Source: three-view drawing plus pictorial views. Frame: mm from the lowest corner of the part. A direction names the side the tool comes from. Round coordinates to 2 decimals unless told otherwise and drop trailing zeros. Write each loop counter-clockwise with the first axis right and the second up, starting at its lowest first coordinate (ties: lowest second). Pieces come first, ordered by that corner, then holes.
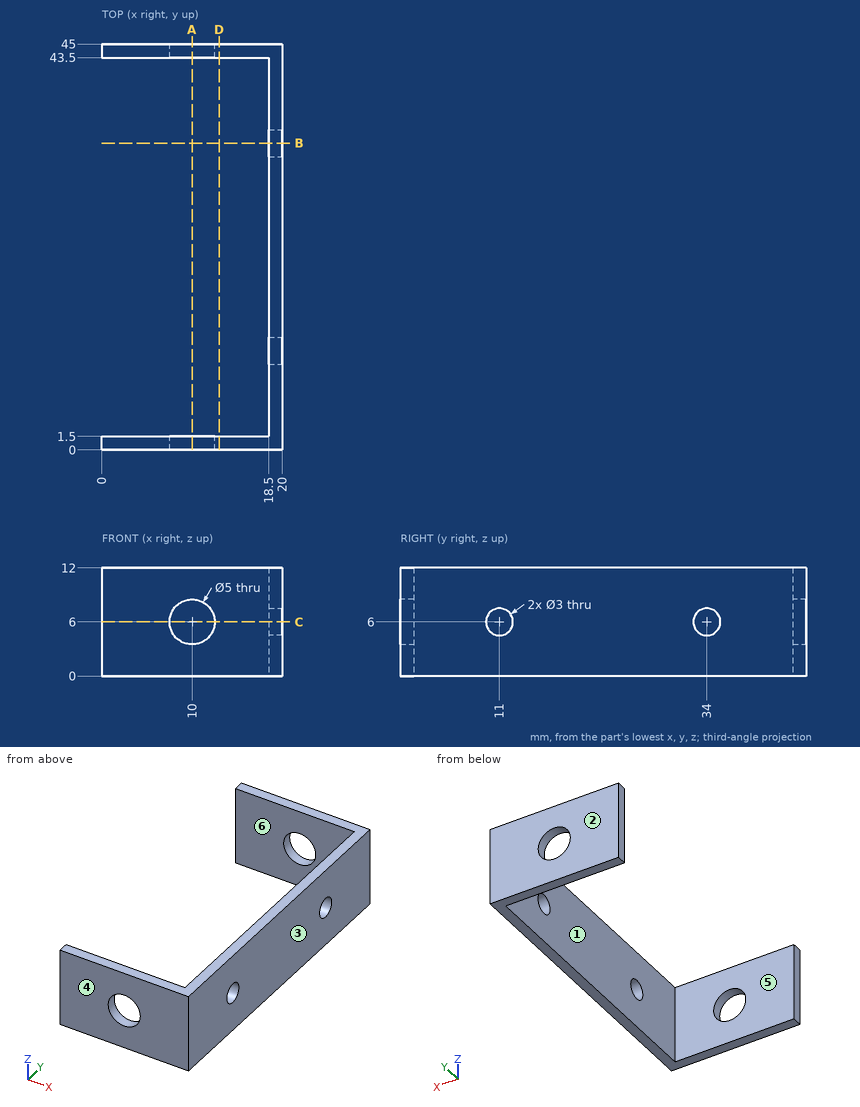
1) Draft query along Y for the marked faces 3, 4, 5 and 6. Return one class per face: pulls with the +Y half, pulls with the -Y half, needs draft (parallel to the pull), parting line crosses it, or undercut.
2) Section C-C on z = 6. Output: boundary loops of the cut face in (x, y), plus the area to 3 significant figures.
3) First-contact query: P1, Ø3.5, axis at y = 13, z = 7, coming from the -X side. Flat tip, straight axial feed; report the tip coordinate or a pass-through.
4) Section A-A on x = 10. Output: boundary loops of the cut face in (y, z).
5) Reachability of the marked faces 1 and 2 from +Z, -Z, +X, -X, +Y, -Y: full face, straight path, thin tool, end or side. Return the list, or none.
6) Line query: probe 1 along Y at (x, z) = (19.6, 6); probe 2 along Y at (x, z) = (8, 0.75); probe 3 along X at (y, z) = (0.5, 6). Output: solid intervals per line, ascending.
7) Section D-D on x = 13. Output: boundary loops of the cut face in (y, z).
8) Section B-B on y = 34. Output: boundary loops of the cut face in (x, z).
Filled in:
1. face 3: needs draft
1. face 4: pulls with the -Y half
1. face 5: undercut
1. face 6: undercut
2. outline: (0, 0) - (7.5, 0) - (7.5, 1.5) - (0, 1.5) - close; (0, 43.5) - (7.5, 43.5) - (7.5, 45) - (0, 45) - close; (12.5, 0) - (20, 0) - (20, 9.5) - (18.5, 9.5) - (18.5, 1.5) - (12.5, 1.5) - close; (12.5, 43.5) - (18.5, 43.5) - (18.5, 35.5) - (20, 35.5) - (20, 45) - (12.5, 45) - close; (18.5, 12.5) - (20, 12.5) - (20, 32.5) - (18.5, 32.5) - close
2. area: 99.0 mm2
3. P1: stops at x = 18.5
4. outline: (0, 0) - (1.5, 0) - (1.5, 3.5) - (0, 3.5) - close; (0, 8.5) - (1.5, 8.5) - (1.5, 12) - (0, 12) - close; (43.5, 0) - (45, 0) - (45, 3.5) - (43.5, 3.5) - close; (43.5, 8.5) - (45, 8.5) - (45, 12) - (43.5, 12) - close
5. face 1: +Z, -Z, -X
5. face 2: +Z, -Z, +X, -X, +Y
6. probe 1: y = 0 to 9.5, 12.5 to 32.5, 35.5 to 45
6. probe 2: y = 0 to 1.5, 43.5 to 45
6. probe 3: x = 0 to 7.5, 12.5 to 20
7. outline: (0, 0) - (1.5, 0) - (1.5, 12) - (0, 12) - close; (43.5, 0) - (45, 0) - (45, 12) - (43.5, 12) - close
8. outline: (18.5, 0) - (20, 0) - (20, 4.5) - (18.5, 4.5) - close; (18.5, 7.5) - (20, 7.5) - (20, 12) - (18.5, 12) - close
